Geometry check sheet. Reference: the model listing, model coordinates, mm. A direction names the side the tool comes from. Coordinates: 2 decimals unless noted, no trailing zeros. Order: outer loops, then holes, each group sorted by start corner. A loop starts at its lowest first (then second) coordinate and runs counter-clockwise, first axis right, second up. Notation, with made-up numbers: (19, 45.5) - (69, 45.5) arc R36 cw to (69, 81.5) - close; hole circle Ø11 at (74, 83.5). An arc over 180 degrees is marked (long way). Put each result on its own line as item: value.
from build123d import *

# Parameters (mm, degrees)
SKETCH1_W                                           = 22.5
SKETCH1_H                                           = 17
SKETCH1_H_2                                         = 25
BOSS_EXTRUDE1_DEPTH                                 = 5
SKETCH1_3_W                                         = 22.5
SKETCH1_3_H                                         = 4
BOSS_EXTRUDE2_DEPTH                                 = 13.5
CBORE_FOR_M2_HEX_SOCKET_HEAD_CAP_SCREW1_D           = 2.4
CBORE_FOR_M2_HEX_SOCKET_HEAD_CAP_SCREW1_CBORE_D     = 4.4
CBORE_FOR_M2_HEX_SOCKET_HEAD_CAP_SCREW1_CBORE_DEPTH = 2.4
BOSS_EXTRUDE3_DEPTH                                 = 5
SKETCH1_4_W                                         = 22.5
SKETCH1_4_H                                         = 4
BOSS_EXTRUDE4_DEPTH                                 = 7.5


with BuildPart() as part:
    # Sketch1 → Boss-Extrude1 (new body)
    with BuildSketch(Plane(origin=(0, 0, 0), x_dir=(1, 0, 0), z_dir=(0, 1, 0))):
        Rectangle(SKETCH1_W, SKETCH1_H)
        Rectangle(SKETCH1_W, SKETCH1_H_2)
    extrude(amount=BOSS_EXTRUDE1_DEPTH)

    # Sketch1<3> → Boss-Extrude2 (add)
    with BuildSketch(Plane(origin=(0, 0, 0), x_dir=(1, 0, 0), z_dir=(0, 1, 0))):
        with Locations((0, 10.5)):
            Rectangle(SKETCH1_3_W, SKETCH1_3_H)
    extrude(amount=-BOSS_EXTRUDE2_DEPTH)

    # CBORE for M2 Hex Socket Head Cap Screw1 (through all)
    with Locations(Plane(origin=(0, 5, 0), x_dir=(1, 0, 0), z_dir=(0, 1, 0))):
        with Locations((-4, -6), (4, 6), (-4, 6), (4, -6)):
            CounterBoreHole(CBORE_FOR_M2_HEX_SOCKET_HEAD_CAP_SCREW1_D / 2, CBORE_FOR_M2_HEX_SOCKET_HEAD_CAP_SCREW1_CBORE_D / 2, CBORE_FOR_M2_HEX_SOCKET_HEAD_CAP_SCREW1_CBORE_DEPTH)

    # Sketch5 → Boss-Extrude3 (add)
    with BuildSketch(Plane.XZ.offset(13.5)):
        Polygon((-11.25, -3), (-11.25, -8.5), (11.25, -8.5), (11.25, -12.5), (41.25, -12.5), (41.25, -3), align=None)
    extrude(amount=-BOSS_EXTRUDE3_DEPTH)

    # Sketch1<4> → Boss-Extrude4 (add)
    with BuildSketch(Plane(origin=(0, 0, 0), x_dir=(1, 0, 0), z_dir=(0, 1, 0))):
        with Locations((0, -10.5)):
            Rectangle(SKETCH1_4_W, SKETCH1_4_H)
    extrude(amount=-BOSS_EXTRUDE4_DEPTH)


solid = part.part
Q1. Section check A-A on x = 4. Record the boundary of the cut face in (y, z), then the cut area to 3 significant figures.
Answer block:
outline: (-13.5, -12.5) - (5, -12.5) - (5, -8.2) - (2.6, -8.2) - (2.6, -7.2) - (0, -7.2) - (0, -8.5) - (-8.5, -8.5) - (-8.5, -3) - (-13.5, -3) - close; (-7.5, 8.5) - (0, 8.5) - (0, 7.2) - (2.6, 7.2) - (2.6, 8.2) - (5, 8.2) - (5, 12.5) - (-7.5, 12.5) - close; (0, -4.8) - (2.6, -4.8) - (2.6, -3.8) - (5, -3.8) - (5, 3.8) - (2.6, 3.8) - (2.6, 4.8) - (0, 4.8) - close
area: 203 mm^2
Q2. Access from +Z, -Z, +X, -X, +Y, -Y to the whole of each face (thin tool, end or side, straight path). Record for faces 4 (the cylindrical face through (5.183, 3.817, -7.855)), 5 (the flat face through (0, -4, 8.5)), 6 (the flat face through (15, -11, -3)).
Answer block:
face 4: +Y
face 5: +X, -X, -Y
face 6: +Z, +X, -X, -Y
Q3. Draft check along X on faces 1 (the flat face through (0, -4, -8.5)), 2 (the flat face through (5, 2.6, 7)), 3 (the flat face through (-11.25, 2, 0)). Enter one of: pulls with the +X half, pulls with the -X half, needs draft (parallel to the pull), parting line crosses it, or undercut.
Answer block:
face 1: needs draft
face 2: undercut
face 3: pulls with the -X half
Q4. Thickness scan on L1, parallel to Z at x = -4, y = 4.25; L2, parallel to Y at x = -8, z = -5.5; L3, parallel to X at y = 1.55, z = 6. Record the ranges inside material, lowest first. Write a range as [from, to].
Answer block:
L1: z = [-12.5, -8.2], [-3.8, 3.8], [8.2, 12.5]
L2: y = [-13.5, -8.5], [0, 5]
L3: x = [-11.25, -5.2], [-2.8, 2.8], [5.2, 11.25]
Q5. Section check B-B on z = -6. Record the boundary of the cut face in (x, y), then the cut area to 3 significant figures.
Answer block:
outline: (-11.25, -13.5) - (41.25, -13.5) - (41.25, -8.5) - (-11.25, -8.5) - close; (-11.25, 0) - (-5.2, 0) - (-5.2, 2.6) - (-6.2, 2.6) - (-6.2, 5) - (-11.25, 5) - close; (-2.8, 0) - (2.8, 0) - (2.8, 2.6) - (1.8, 2.6) - (1.8, 5) - (-1.8, 5) - (-1.8, 2.6) - (-2.8, 2.6) - close; (5.2, 0) - (11.25, 0) - (11.25, 5) - (6.2, 5) - (6.2, 2.6) - (5.2, 2.6) - close
area: 341 mm^2
Q6. Depth check by flat-ended pin: pin 1 Ø4 at (y, z) = (-4, -9) entering from +X; pin 2 Ø5 at (x, z) = (16.5, -6) entering from +Y; pin 3 Ø5.5 at (x, z) = (-4, -6) entering from +Y; pin 4 Ø2.5 at (x, y) = (7.5, -10) entering from +Z. Enter the tip coordinate at first touch or a pass-through.
Answer block:
pin 1: stops at x = 11.25
pin 2: stops at y = -8.5
pin 3: stops at y = 5
pin 4: stops at z = -3
Q7. Section check D-D on y = -5. Record the boundary of the cut face in (x, z).
Answer block:
outline: (-11.25, -12.5) - (11.25, -12.5) - (11.25, -8.5) - (-11.25, -8.5) - close; (-11.25, 8.5) - (11.25, 8.5) - (11.25, 12.5) - (-11.25, 12.5) - close
Q8. Section check C-C on y = 0.5. Record the boundary of the cut face in (x, z).
Answer block:
outline: (-11.25, -12.5) - (11.25, -12.5) - (11.25, 12.5) - (-11.25, 12.5) - close; hole circle Ø2.4 at (-4, -6); hole circle Ø2.4 at (-4, 6); hole circle Ø2.4 at (4, -6); hole circle Ø2.4 at (4, 6)
